Check sheet for the modelled part. Datum: model origin and axes. Units: mm. Round coordinates to 2 decimals unless told otherwise and drop trailing zeros. Loops run counter-clockwise (first coordinate to the right, second up) from the corner with the lowest first, then second, coordinate; pieces in that order, holes last. Notation, with made-up numbers: (17.5, 67.5) -> (60.5, 67.5) arc R27 cw to (60.5, 102.5) -> close; hole circle Ø10 at (22.25, 43.5). An arc over 180 degrees is marked (long way). Return JSON: item names as keys, results as strings.
from build123d import *

# Parameters (mm, degrees)
SCHIZZO1_R                   = 2.1
ESTRUSIONE_ESTRUSIONE1_DEPTH = 3
SMUSSO1_SIZE                 = 2
ESTRUSIONE_ESTRUSIONE2_DEPTH = 50
SCHIZZO3_R                   = 2.1
TAGLIO_ESTRUSIONE1_DEPTH     = 10
RACCORDO1_R                  = 5
TAGLIO_ESTRUSIONE3_REACH     = 77.873
SCHIZZO5_R                   = 4.5


with BuildPart() as part:
    # Schizzo1 → Estrusione-Estrusione1 (new body)
    with BuildSketch(Plane.XY):
        Polygon((0, 71.847389048), (25, 71.847389048), (25, 12.801854913), (0, 12.801854913), (-25, 12.801854913), (-25, 71.847389048), align=None)
        with Locations((18.75, 57.086005514)):
            Circle(SCHIZZO1_R, mode=Mode.SUBTRACT)
        with Locations((18.75, 27.563238447)):
            Circle(SCHIZZO1_R, mode=Mode.SUBTRACT)
        with Locations(Location((-18.75, 27.563238447, 0), (0, 0, 180))):
            Circle(SCHIZZO1_R, mode=Mode.SUBTRACT)
        with Locations(Location((-18.75, 57.086005514, 0), (0, 0, 180))):
            Circle(SCHIZZO1_R, mode=Mode.SUBTRACT)
        with Locations((0, 58.89473309)):
            Circle(SCHIZZO1_R, mode=Mode.SUBTRACT)
        with Locations((0, 31.80362551)):
            Circle(SCHIZZO1_R, mode=Mode.SUBTRACT)
    extrude(amount=ESTRUSIONE_ESTRUSIONE1_DEPTH)

    # Smusso1
    smusso1_edges = [part.edges().sort_by_distance(p)[0] for p in [
        (-2.1, 58.89473309, 0),
        (-2.1, 31.80362551, 0),
    ]]
    chamfer(smusso1_edges, length=SMUSSO1_SIZE)

    # Schizzo2 → Estrusione-Estrusione2 (add)
    with BuildSketch(Plane(origin=(25, 0, 0), x_dir=(0, 0, -1), z_dir=(1, 0, 0))):
        Polygon((-3, 71.847389048), (-8.165814869, 12.801854913), (-3, 12.801854913), align=None)
    extrude(amount=-ESTRUSIONE_ESTRUSIONE2_DEPTH)

    # Schizzo3 → Taglio-Estrusione1 (cut)
    with BuildSketch(Plane(origin=(0, 0, 3), x_dir=(-1, 0, 0), z_dir=(0, 0, -1))):
        with Locations((18.75, 27.563238447)):
            Circle(SCHIZZO3_R)
        with Locations((18.75, 57.086005514)):
            Circle(SCHIZZO3_R)
        with Locations(Location((-18.75, 57.086005514, 0), (0, 0, 90))):
            Circle(SCHIZZO3_R)
        with Locations(Location((-18.75, 27.563238447, 0), (0, 0, 90))):
            Circle(SCHIZZO3_R)
        with Locations(Location((0, 31.80362551, 0), (0, 0, 90))):
            Circle(SCHIZZO3_R)
        with Locations(Location((0, 58.89473309, 0), (0, 0, 90))):
            Circle(SCHIZZO3_R)
    extrude(amount=-TAGLIO_ESTRUSIONE1_DEPTH, mode=Mode.SUBTRACT)

    # Raccordo1
    raccordo1_edges = [part.edges().sort_by_distance(p)[0] for p in [
        (25, 71.847389048, 1.5),
        (25, 12.801854913, 4.082907434),
        (-25, 12.801854913, 4.082907434),
        (-25, 71.847389048, 1.5),
    ]]
    fillet(raccordo1_edges, radius=RACCORDO1_R)

    # Taglio-Estrusione3: up to this plane
    taglio_estrusione3_end = Plane(origin=(0, 0, 3.5), z_dir=(0, 0, 1))
    # Schizzo5 → Taglio-Estrusione3 (cut, up to the surface)
    with BuildSketch(Plane(origin=(0, 0.806233906, 9.215295719), x_dir=(1, 0, 0), z_dir=(0, 0.08715574274765137, 0.9961946980917462)), mode=Mode.PRIVATE) as taglio_estrusione3_sk1:
        with Locations(Location((-18.75, 56.494751192, 0), (0, 0, 270))):
            Circle(SCHIZZO5_R)
    taglio_estrusione3_tool1 = split(extrude(taglio_estrusione3_sk1.sketch, amount=-TAGLIO_ESTRUSIONE3_REACH, mode=Mode.PRIVATE), bisect_by=taglio_estrusione3_end, keep=Keep.BOTH, mode=Mode.PRIVATE)
    add(taglio_estrusione3_tool1.solids().sort_by_distance((-18.75, 57.086006, 4.291454))[0], mode=Mode.SUBTRACT)
    # Schizzo5 → Taglio-Estrusione3 (cut, up to the surface)
    with BuildSketch(Plane(origin=(0, 0.806233906, 9.215295719), x_dir=(1, 0, 0), z_dir=(0, 0.08715574274765137, 0.9961946980917462)), mode=Mode.PRIVATE) as taglio_estrusione3_sk2:
        with Locations(Location((18.75, 56.494751192, 0), (0, 0, 270))):
            Circle(SCHIZZO5_R)
    taglio_estrusione3_tool2 = split(extrude(taglio_estrusione3_sk2.sketch, amount=-TAGLIO_ESTRUSIONE3_REACH, mode=Mode.PRIVATE), bisect_by=taglio_estrusione3_end, keep=Keep.BOTH, mode=Mode.PRIVATE)
    add(taglio_estrusione3_tool2.solids().sort_by_distance((18.75, 57.086006, 4.291454))[0], mode=Mode.SUBTRACT)
    # Schizzo5 → Taglio-Estrusione3 (cut, up to the surface)
    with BuildSketch(Plane(origin=(0, 0.806233906, 9.215295719), x_dir=(1, 0, 0), z_dir=(0, 0.08715574274765137, 0.9961946980917462)), mode=Mode.PRIVATE) as taglio_estrusione3_sk3:
        with Locations(Location((18.75, 26.859211951, 0), (0, 0, 270))):
            Circle(SCHIZZO5_R)
    taglio_estrusione3_tool3 = split(extrude(taglio_estrusione3_sk3.sketch, amount=-TAGLIO_ESTRUSIONE3_REACH, mode=Mode.PRIVATE), bisect_by=taglio_estrusione3_end, keep=Keep.BOTH, mode=Mode.PRIVATE)
    add(taglio_estrusione3_tool3.solids().sort_by_distance((18.75, 27.563238, 6.874361))[0], mode=Mode.SUBTRACT)
    # Schizzo5 → Taglio-Estrusione3 (cut, up to the surface)
    with BuildSketch(Plane(origin=(0, 0.806233906, 9.215295719), x_dir=(1, 0, 0), z_dir=(0, 0.08715574274765137, 0.9961946980917462)), mode=Mode.PRIVATE) as taglio_estrusione3_sk4:
        with Locations(Location((-18.75, 26.859211951, 0), (0, 0, 270))):
            Circle(SCHIZZO5_R)
    taglio_estrusione3_tool4 = split(extrude(taglio_estrusione3_sk4.sketch, amount=-TAGLIO_ESTRUSIONE3_REACH, mode=Mode.PRIVATE), bisect_by=taglio_estrusione3_end, keep=Keep.BOTH, mode=Mode.PRIVATE)
    add(taglio_estrusione3_tool4.solids().sort_by_distance((-18.75, 27.563238, 6.874361))[0], mode=Mode.SUBTRACT)


solid = part.part
Q1. Section check A-A (x = 18.75). Record the boundary of the cut face in (y, z), then the cut area to 3 significant figures.
Results list:
{"outline": "(12.8, 0) -> (25.46, 0) -> (25.46, 3.5) -> (22.75, 3.5) -> (23.08, 7.27) -> (12.8, 8.17) -> close; (29.66, 0) -> (54.99, 0) -> (54.99, 3.5) -> (52.5, 3.5) -> (52.6, 4.68) -> (32.05, 6.48) -> (31.79, 3.5) -> (29.66, 3.5) -> close; (59.19, 0) -> (71.85, 0) -> (71.85, 3) -> (61.57, 3.9) -> (61.53, 3.5) -> (59.19, 3.5) -> close", "area": "263 mm^2"}
Q2. Go/stop test with flat-tipped pins: pin 1 (2.5 mm diameter, centred on x = 0, y = 58.89, fed in from +Z); pin 2 (4.5 mm diameter, centred on x = -19, y = 28, fed in from +Z); pin 3 (6.5 mm diameter, centred on x = 0, y = 31.8, fed in from -Z). Record where each tip stops, or that it passes through.
Results list:
{"pin 1": "through", "pin 2": "z = 3.5", "pin 3": "z = 0.85"}
Q3. Section check C-C (y = 67.5). Record the boundary of the cut face in (x, z), then the cut area to 3 significant figures.
Results list:
{"outline": "(-24.96, 0) -> (24.96, 0) -> (24.96, 3.38) -> (-24.96, 3.38) -> close", "area": "169 mm^2"}
Q4. Section check D-D (x = -6.5). Record the boundary of the cut face in (y, z).
Results list:
{"outline": "(12.8, 0) -> (71.85, 0) -> (71.85, 3) -> (12.8, 8.17) -> close"}
Q5. Section check B-B (x = -15). Record the boundary of the cut face in (y, z) (3 decimals), then the cut area to 3 significant figures.
Results list:
{"outline": "(12.802, 0) -> (71.847, 0) -> (71.847, 3) -> (59.564, 4.075) -> (59.514, 3.5) -> (54.52, 3.5) -> (54.608, 4.508) -> (30.041, 6.658) -> (29.765, 3.5) -> (24.771, 3.5) -> (25.085, 7.091) -> (12.802, 8.166) -> close", "area": "309 mm^2"}
Q6. Draft check along X on faces 1 (the flat face through (-25, 37, 3)), 2 (the conical face through (-0.482, 56.723, 1.875)), 3 (the flat face through (-19, 25, 3.5)), 4 (the flat face through (25, 37, 3)). Enter one of: released by +X, released by -X, zero draft, split by the parting line, or undercut.
Results list:
{"face 1": "released by -X", "face 2": "undercut", "face 3": "undercut", "face 4": "released by +X"}
Q7. Material ranges on line 1 (Y direction, x = 18.75, z = 1.2); line 2 (X direction, y = 26.5, z = 2); line 3 (Y direction, x = 17.5, z = 7), recorded low to high.
Results list:
{"line 1": "12.8 to 25.46, 29.66 to 54.99, 59.19 to 71.85", "line 2": "-25 to -20.56, -16.94 to 16.94, 20.56 to 25", "line 3": "12.8 to 23.23"}
